from build123d import *

# Parameters (mm, degrees)
BOSS_EXTRUDE3_DEPTH = 120
BOSS_EXTRUDE4_DEPTH = 2
BOSS_EXTRUDE5_DEPTH = 15
SKETCH8_W           = 16
SKETCH8_H           = 13
CUT_EXTRUDE2_DEPTH  = 15


with BuildPart() as part:
    # Sketch4 → Boss-Extrude3 (new body)
    with BuildSketch(Plane(origin=(0, 0, 0), x_dir=(1, 0, 0), z_dir=(0, 1, 0))):
        with BuildLine():
            Line((-80, -192.509889923), (-80, -206.5))
            Line((-80, -206.5), (80, -206.5))
            Line((80, -206.5), (80, -192.509889923))
            add(Edge.make_bspline(
                [(-80, -192.509889923), (-72.106688699, -194.086619514), (-45.4407372, -198.624917909), (0, -201.8200332), (45.4407372, -198.624917909), (72.106688699, -194.086619514), (80, -192.509889923)],
                knots=[0.498587518, 0.498587518, 0.498587518, 0.498587518, 0.499005631, 0.5, 0.500994369, 0.501412482, 0.501412482, 0.501412482, 0.501412482], degree=3))
        make_face()
    extrude(amount=BOSS_EXTRUDE3_DEPTH)

    # Sketch6 → Boss-Extrude4 (add)
    with BuildSketch(Plane.XZ):
        with BuildLine():
            Line((10, 0), (10, 206.5))
            Line((10, 206.5), (-10, 206.5))
            Line((-10, 206.5), (-10, 0))
            ThreePointArc((-10, 0), (0, -10), (10, 0))
        make_face()
    extrude(amount=BOSS_EXTRUDE4_DEPTH)

    # Sketch7 → Boss-Extrude5 (add)
    with BuildSketch(Plane.XZ.offset(2)):
        with BuildLine():
            Line((10, 0), (10, 206.5))
            Line((10, 206.5), (-10, 206.5))
            Line((-10, 206.5), (-10, 0))
            ThreePointArc((-10, 0), (0, -10), (10, 0))
        make_face()
        with BuildLine():
            Line((8, 0), (8, 204.5))
            Line((8, 204.5), (-8, 204.5))
            Line((-8, 204.5), (-8, 0))
            ThreePointArc((-8, 0), (0, -8), (8, 0))
        make_face(mode=Mode.SUBTRACT)
    extrude(amount=BOSS_EXTRUDE5_DEPTH)

    # Sketch8 → Cut-Extrude2 (cut)
    with BuildSketch(Plane.XY.offset(206.5)):
        with Locations((0, -8.5)):
            Rectangle(SKETCH8_W, SKETCH8_H)
    extrude(amount=-CUT_EXTRUDE2_DEPTH, mode=Mode.SUBTRACT)


solid = part.part
Input: part model. Units: mm. Frame: model coordinates. A direction names the side the tool comes from. Coordinates: 2 decimals unless noted, no trailing zeros. Loops run counter-clockwise (first coordinate to the right, second up) from the corner with the lowest first, then second, coordinate; pieces in that order, holes last.
Q1. Material intervals for line 1 (Y direction, x = -4.5, z = 193); line 2 (Y direction, x = -9, z = 97.5); line 3 (Z direction, x = 9, y = 33), sorted ascending.
Q2. Set-up query: faces 1 (the face through (52, 0, 203)), 2 (the face through (80, 59, 200)). Return all of +Z, -Z, +X, -X, +Y, -Y with unobstructed straight access to the full face (end or side cutting, diameter ignored); none if empty.
Q3. Contact query for flat-ended pins moving along their axis: pin 1 (8.5 mm diameter, centred on y = -8.5, z = 111, fed in from +X); pin 2 (4 mm diameter, centred on x = 32, y = 27.5, fed in from -Z); pin 3 (8 mm diameter, centred on x = -1.5, z = 136.5, fed in from -Y). Output: stop coordinate, or through.
Q4. Cut plane A-A (z = 47.5). Output: boundary loops of the cut face in (x, y), then the cut area to 3 significant figures.
Q5. Draft query along X for faces 3 (the face through (-53, 0, 201)), 4 (the face through (-80, 59, 199)), 5 (the face through (-8, -9, 105)). Return one class per face: +X half, -X half, draft (parallel to the pull), parting line (faces both ways), or undercut.
Working result:
1. line 1: y = -2 to 0
1. line 2: y = -17 to 0
1. line 3: z = 200.4 to 206.5
2. face 1: +Z, -Z, +X, -Y
2. face 2: +Z, -Z, +X, +Y, -Y
3. pin 1: stops at x = 10
3. pin 2: stops at z = 199.06
3. pin 3: stops at y = -2
4. outline: (-10, -17) - (-8, -17) - (-8, -2) - (8, -2) - (8, -17) - (10, -17) - (10, 0) - (-10, 0) - close
4. area: 100 mm2
5. face 3: draft
5. face 4: -X half
5. face 5: undercut
